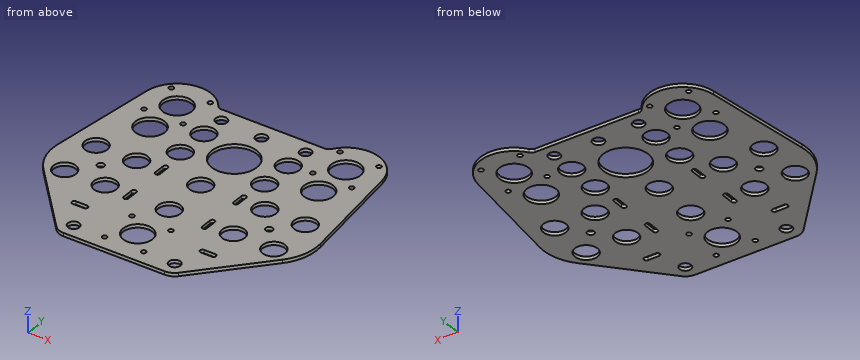
from build123d import *

# Parameters (mm, degrees)
MODEL_R             = 2.1
MODEL_R_2           = 13
MODEL_R_3           = 3.1
MODEL_R_4           = 10
MODEL_R_5           = 5.1
MODEL_R_6           = 20
BOSS_EXTRUDE1_DEPTH = 3


with BuildPart() as part:
    # Model → Boss-Extrude1 (new body)
    with BuildSketch(Plane.XY):
        with BuildLine():
            Line((-44.9, -112.113099849), (0, -112.113099849))
            Line((0, -112.113099849), (44.9, -112.113099849))
            ThreePointArc((44.9, -112.113099849), (50.059264201, -111.015645267), (54.325169295, -107.913312696))
            Line((54.325169295, -107.913312696), (106.229152519, -50.197615742))
            ThreePointArc((106.229152519, -50.197615742), (115.069026633, -34.701709967), (116.679519982, -16.934527261))
            Line((116.679519982, -16.934527261), (104.771085702, 78.90999671))
            ThreePointArc((104.771085702, 78.90999671), (82.034748438, 104.374560561), (50.189310486, 92.0760596))
            ThreePointArc((50.189310486, 92.0760596), (48.393618278, 90.467952157), (46.054195567, 89.886900151))
            Line((46.054195567, 89.886900151), (0, 89.886900151))
            Line((0, 89.886900151), (-46.054195567, 89.886900151))
            ThreePointArc((-46.054195567, 89.886900151), (-48.393618278, 90.467952157), (-50.189310486, 92.0760596))
            ThreePointArc((-50.189310486, 92.0760596), (-82.034748438, 104.374560561), (-104.771085702, 78.90999671))
            Line((-104.771085702, 78.90999671), (-116.679519982, -16.934527261))
            ThreePointArc((-116.679519982, -16.934527261), (-115.069026633, -34.701709967), (-106.229152519, -50.197615742))
            Line((-106.229152519, -50.197615742), (-54.325169295, -107.913312696))
            ThreePointArc((-54.325169295, -107.913312696), (-50.059264201, -111.015645267), (-44.9, -112.113099849))
        make_face()
        with Locations((17.324116139, -99.437215988)):
            Circle(MODEL_R, mode=Mode.SUBTRACT)
        with Locations((-17.324116139, -64.78898371)):
            Circle(MODEL_R, mode=Mode.SUBTRACT)
        with Locations((-92.324116139, 57.886900151)):
            Circle(MODEL_R, mode=Mode.SUBTRACT)
        with Locations((-57.675883861, 92.535132429)):
            Circle(MODEL_R, mode=Mode.SUBTRACT)
        with Locations((0, -82.113099849)):
            Circle(MODEL_R_2, mode=Mode.SUBTRACT)
        with Locations((-75, 75.21101629)):
            Circle(MODEL_R_2, mode=Mode.SUBTRACT)
        with Locations((-92.324116139, 92.535132429)):
            Circle(MODEL_R, mode=Mode.SUBTRACT)
        with Locations((-57.675883861, 57.886900151)):
            Circle(MODEL_R, mode=Mode.SUBTRACT)
        with Locations((17.324116139, -64.78898371)):
            Circle(MODEL_R, mode=Mode.SUBTRACT)
        with Locations((-17.324116139, -99.437215988)):
            Circle(MODEL_R, mode=Mode.SUBTRACT)
        with Locations((-75, -22.113099849)):
            Circle(MODEL_R_3, mode=Mode.SUBTRACT)
        with Locations((-57, -2.113099849)):
            Circle(MODEL_R_4, mode=Mode.SUBTRACT)
        with Locations((-57, -42.113099849)):
            Circle(MODEL_R_4, mode=Mode.SUBTRACT)
        with Locations((-93, -2.113099849)):
            Circle(MODEL_R_4, mode=Mode.SUBTRACT)
        with Locations((-93, -42.113099849)):
            Circle(MODEL_R_4, mode=Mode.SUBTRACT)
        with Locations((-44.9, -99.437215988)):
            Circle(MODEL_R_5, mode=Mode.SUBTRACT)
        with Locations((75, -22.113099849)):
            Circle(MODEL_R_3, mode=Mode.SUBTRACT)
        with Locations((57, -2.113099849)):
            Circle(MODEL_R_4, mode=Mode.SUBTRACT)
        with Locations((57, -42.113099849)):
            Circle(MODEL_R_4, mode=Mode.SUBTRACT)
        with Locations((93, -2.113099849)):
            Circle(MODEL_R_4, mode=Mode.SUBTRACT)
        with Locations((93, -42.113099849)):
            Circle(MODEL_R_4, mode=Mode.SUBTRACT)
        with Locations((44.9, -99.437215988)):
            Circle(MODEL_R_5, mode=Mode.SUBTRACT)
        with Locations((0, 75.21101629)):
            Circle(MODEL_R_5, mode=Mode.SUBTRACT)
        with Locations((0, -2.113099849)):
            Circle(MODEL_R_4, mode=Mode.SUBTRACT)
        with Locations((0, -42.113099849)):
            Circle(MODEL_R_4, mode=Mode.SUBTRACT)
        with Locations((0, 40.562784012)):
            Circle(MODEL_R_6, mode=Mode.SUBTRACT)
        with Locations((-37.5, 55.562784012)):
            Circle(MODEL_R_4, mode=Mode.SUBTRACT)
        with Locations((-37.5, 25.562784012)):
            Circle(MODEL_R_4, mode=Mode.SUBTRACT)
        with Locations((37.5, 55.562784012)):
            Circle(MODEL_R_4, mode=Mode.SUBTRACT)
        with Locations((37.5, 25.562784012)):
            Circle(MODEL_R_4, mode=Mode.SUBTRACT)
        with Locations((57.675883861, 57.886900151)):
            Circle(MODEL_R, mode=Mode.SUBTRACT)
        with Locations((92.324116139, 92.535132429)):
            Circle(MODEL_R, mode=Mode.SUBTRACT)
        with Locations((75, 75.21101629)):
            Circle(MODEL_R_2, mode=Mode.SUBTRACT)
        with Locations((57.675883861, 92.535132429)):
            Circle(MODEL_R, mode=Mode.SUBTRACT)
        with Locations((92.324116139, 57.886900151)):
            Circle(MODEL_R, mode=Mode.SUBTRACT)
        with Locations((-75, 40.688174024)):
            Circle(MODEL_R_2, mode=Mode.SUBTRACT)
        with Locations((75, 40.562784012)):
            Circle(MODEL_R_2, mode=Mode.SUBTRACT)
        with Locations((-37.5, 77.724842082)):
            Circle(MODEL_R_5, mode=Mode.SUBTRACT)
        with Locations((37.5, 77.724842082)):
            Circle(MODEL_R_5, mode=Mode.SUBTRACT)
        with BuildLine():
            Line((-37, 2.886900151), (-37, -7.113099849))
            ThreePointArc((-37, -7.113099849), (-34.9, -9.213099849), (-32.8, -7.113099849))
            Line((-32.8, -7.113099849), (-32.8, 2.886900151))
            ThreePointArc((-32.8, 2.886900151), (-34.9, 4.986900151), (-37, 2.886900151))
        make_face(mode=Mode.SUBTRACT)
        with BuildLine():
            Line((-37, -37.113099849), (-37, -47.113099849))
            ThreePointArc((-37, -47.113099849), (-34.9, -49.213099849), (-32.8, -47.113099849))
            Line((-32.8, -47.113099849), (-32.8, -37.113099849))
            ThreePointArc((-32.8, -37.113099849), (-34.9, -35.013099849), (-37, -37.113099849))
        make_face(mode=Mode.SUBTRACT)
        with BuildLine():
            Line((37, 2.886900151), (37, -7.113099849))
            ThreePointArc((37, -7.113099849), (34.9, -9.213099849), (32.8, -7.113099849))
            Line((32.8, -7.113099849), (32.8, 2.886900151))
            ThreePointArc((32.8, 2.886900151), (34.9, 4.986900151), (37, 2.886900151))
        make_face(mode=Mode.SUBTRACT)
        with BuildLine():
            Line((37, -37.113099849), (37, -47.113099849))
            ThreePointArc((37, -47.113099849), (34.9, -49.213099849), (32.8, -47.113099849))
            Line((32.8, -47.113099849), (32.8, -37.113099849))
            ThreePointArc((32.8, -37.113099849), (34.9, -35.013099849), (37, -37.113099849))
        make_face(mode=Mode.SUBTRACT)
        with BuildLine():
            Line((-62, -72.113099849), (-52, -72.113099849))
            ThreePointArc((-52, -72.113099849), (-49.9, -74.213099849), (-52, -76.313099849))
            Line((-52, -76.313099849), (-62, -76.313099849))
            ThreePointArc((-62, -76.313099849), (-64.1, -74.213099849), (-62, -72.113099849))
        make_face(mode=Mode.SUBTRACT)
        with BuildLine():
            Line((62, -72.113099849), (52, -72.113099849))
            ThreePointArc((52, -72.113099849), (49.9, -74.213099849), (52, -76.313099849))
            Line((52, -76.313099849), (62, -76.313099849))
            ThreePointArc((62, -76.313099849), (64.1, -74.213099849), (62, -72.113099849))
        make_face(mode=Mode.SUBTRACT)
    extrude(amount=BOSS_EXTRUDE1_DEPTH)


solid = part.part
Geometry check sheet. Reference: the model listing, model coordinates, mm. Round coordinates to 2 decimals unless told otherwise and drop trailing zeros. Order: outer loops, then holes, each group sorted by start corner. A loop starts at its lowest first (then second) coordinate and runs counter-clockwise, first axis right, second up. Notation, with made-up numbers: (60, 32) - (75, 32) arc R23 cw to (75, 62) - close; hole circle Ø1 at (87.5, 0.25). An arc over 180 degrees is marked (long way). One line per question, with ' | ' between items. Start each with the question number.
(1) Sectioned sample at D-D on z = 2.3. Count the separate pieces of the cut face and the enclosed holes in it, and give its area (3 significant figures).
(2) Sectioned sample at A-A on x = -75. Record the cut outline in (y, z), and give its area (3 significant figures).
(3) Thickness scan on L1, parallel to Y at x = 0, z = 0.9; L2, parallel to X at y = -81.5, z = 0.85; L3, parallel to Y at x = -87, z = 2.5. Record the ranges inside material, lowest first. Write a range as [from, to].
(4) Sectioned sample at B-B on y = 50.5. Record the cut outline in (x, z), and give its area (3 significant figures).
(5) Sectioned sample at C-C on x = -2. Record the cut outline in (y, z).
(6) Depth check by flat-ended pin: pin 1 Ø16 at (x, y) = (-93, -42.11) entering from +Z; pin 2 Ø1.5 at (x, z) = (-92, 0.5) entering from +Y; pin 3 Ø1 at (y, z) = (-36.5, 1) entering from +X; pin 4 Ø16.5 at (x, y) = (-37.5, 77.72) entering from +Z. Enter the tip coordinate at first touch or a pass-through.
Conclusion:
1) separate pieces: 1 | enclosed holes: 45 | area: 32,600 mm2
2) outline: (-84.92, 0) - (-25.21, 0) - (-25.21, 3) - (-84.92, 3) - close; (-19.01, 0) - (27.69, 0) - (27.69, 3) - (-19.01, 3) - close; (53.69, 0) - (62.21, 0) - (62.21, 3) - (53.69, 3) - close; (88.21, 0) - (105.21, 0) - (105.21, 3) - (88.21, 3) - close | area: 396 mm2
3) L1: y = [-112.11, -95.11], [-69.11, -52.11], [-32.11, -12.11], [7.89, 20.56], [60.56, 70.11], [80.31, 89.89] | L2: x = [-78.08, -12.99], [12.99, 78.08] | L3: y = [-71.58, -50.11], [-34.11, -10.11], [5.89, 35.69], [45.69, 70.21], [80.21, 102.71]
4) outline: (-108.3, 0) - (-83.53, 0) - (-83.53, 3) - (-108.3, 3) - close; (-66.47, 0) - (-46.12, 0) - (-46.12, 3) - (-66.47, 3) - close; (-28.88, 0) - (-17.36, 0) - (-17.36, 3) - (-28.88, 3) - close; (17.36, 0) - (28.88, 0) - (28.88, 3) - (17.36, 3) - close; (46.12, 0) - (66.62, 0) - (66.62, 3) - (46.12, 3) - close; (83.38, 0) - (108.3, 0) - (108.3, 3) - (83.38, 3) - close | area: 341 mm2
5) outline: (-112.11, 0) - (-94.96, 0) - (-94.96, 3) - (-112.11, 3) - close; (-69.27, 0) - (-51.91, 0) - (-51.91, 3) - (-69.27, 3) - close; (-32.32, 0) - (-11.91, 0) - (-11.91, 3) - (-32.32, 3) - close; (7.68, 0) - (20.66, 0) - (20.66, 3) - (7.68, 3) - close; (60.46, 0) - (70.52, 0) - (70.52, 3) - (60.46, 3) - close; (79.9, 0) - (89.89, 0) - (89.89, 3) - (79.9, 3) - close
6) pin 1: passes through | pin 2: stops at y = 100.43 | pin 3: stops at x = 114.64 | pin 4: stops at z = 3
